from build123d import *

# Parameters (mm, degrees)
BOSS_EXTRUDE1_DEPTH                  = 3.175
F_1_4_0_25_DIAMETER_HOLE1_D          = 6.35
F_1_4_0_25_DIAMETER_HOLE3_AT_2_COUNT = 2
F_1_4_0_25_DIAMETER_HOLE3_AT_2_PITCH = 25.4
F_1_4_0_25_DIAMETER_HOLE3_AT_3_COUNT = 2
F_1_4_0_25_DIAMETER_HOLE3_AT_3_PITCH = 71.842048969
F_1_4_0_25_DIAMETER_HOLE3_AT_4_COUNT = 2
F_1_4_0_25_DIAMETER_HOLE3_AT_4_PITCH = 91.581002397


with BuildPart() as part:
    # Outline → Boss-Extrude1 (new body)
    with BuildSketch(Plane.XZ.offset(-43.833362877)):
        with BuildLine():
            Line((176.972439461, -654.113339272), (243.430903053, -587.760058499))
            ThreePointArc((243.430903053, -587.760058499), (244.176274012, -585.964597022), (243.433747886, -584.167957177))
            Line((243.433747886, -584.167957177), (231.320007239, -572.035013901))
            ThreePointArc((231.320007239, -572.035013901), (229.524545763, -571.289642942), (227.727905917, -572.032169067))
            Line((227.727905917, -572.032169067), (202.161954847, -597.557657288))
            ThreePointArc((202.161954847, -597.557657288), (175.212357167, -608.695549172), (148.280435018, -597.514984781))
            Line((148.280435018, -597.514984781), (123.155639602, -572.350361691))
            ThreePointArc((123.155639602, -572.350361691), (121.360178125, -571.604990731), (119.56353828, -572.347516857))
            Line((119.56353828, -572.347516857), (107.430595004, -584.461257504))
            ThreePointArc((107.430595004, -584.461257504), (106.685224045, -586.256718981), (107.42775017, -588.053358826))
            Line((107.42775017, -588.053358826), (173.380338139, -654.110494438))
            ThreePointArc((173.380338139, -654.110494438), (175.175799616, -654.855865397), (176.972439461, -654.113339272))
        make_face()
    extrude(amount=BOSS_EXTRUDE1_DEPTH)

    # 1/4 (0.25) Diameter Hole1 (through all)
    with Locations(Plane(origin=(0, 40.658362877, 0), x_dir=(-1, 0, 0), z_dir=(0, -1, 0))):
        with Locations((-175.18563451, 642.437587559), (-193.160365289, 624.491305118), (-157.239352069, 624.46285678)):
            Hole(F_1_4_0_25_DIAMETER_HOLE1_D / 2)

    # Sketch11 → 1/4 (0.25) Diameter Hole3 (revolve, cut)
    with BuildSketch(Plane(origin=(139.293069629, 40.658362877, -606.488126001), x_dir=(0, 0, -1), z_dir=(1, 0, 0))):
        Polygon((0, 0), (0, 3.175), (3.175, 3.175), (3.175, 3.944613268), (6.604, 0), align=None)
    f_1_4_0_25_diameter_hole3 = revolve(axis=Axis((139.293069629, 34.308362877, -606.488126001), (0, 1, 0)), mode=Mode.SUBTRACT)

    # 1/4 (0.25) Diameter Hole3 at 2: 1/4 (0.25) Diameter Hole3 ×2
    with Locations(*[Vector(-0.7065465527738991, 0, 0.7076665660912065) * (i * F_1_4_0_25_DIAMETER_HOLE3_AT_2_PITCH) for i in range(1, F_1_4_0_25_DIAMETER_HOLE3_AT_2_COUNT)]):
        add(f_1_4_0_25_diameter_hole3, mode=Mode.SUBTRACT)

    # 1/4 (0.25) Diameter Hole3 at 3: 1/4 (0.25) Diameter Hole3 ×2
    with Locations(*[Vector(0.9999996863924931, 0, -0.0007919690116880901) * (i * F_1_4_0_25_DIAMETER_HOLE3_AT_3_PITCH) for i in range(1, F_1_4_0_25_DIAMETER_HOLE3_AT_3_COUNT)]):
        add(f_1_4_0_25_diameter_hole3, mode=Mode.SUBTRACT)

    # 1/4 (0.25) Diameter Hole3 at 4: 1/4 (0.25) Diameter Hole3 ×2
    with Locations(*[Vector(0.980735686075181, 0, 0.1953394841260828) * (i * F_1_4_0_25_DIAMETER_HOLE3_AT_4_PITCH) for i in range(1, F_1_4_0_25_DIAMETER_HOLE3_AT_4_COUNT)]):
        add(f_1_4_0_25_diameter_hole3, mode=Mode.SUBTRACT)


solid = part.part
Geometry: final body of the model. Coordinates: model frame, mm. A direction names the side the tool comes from. Give positions to 0.01 mm unless a question says otherwise; leave off trailing zeros. Write each loop counter-clockwise with the first axis right and the second up, starting at its lowest first coordinate (ties: lowest second). Pieces come first, ordered by that corner, then holes.
(1) Cut plane C-C, the plane x = 130. Return loops of the section in (y, z), then the cut area to 3 significant figures.
(2) Cut plane A-A, the plane y = 41.4. Give the number of separate pieces and of enclosed holes in the cut face, then the cut area to 3 significant figures.
(3) Cut plane B-B, the plane z = -641. Return loops of the section in (x, y), then the cut area to 3 significant figures.
(4) Mould query, pull axis Z, two halves, no side actions, for faces 1 (the conical face through (227.903, 43.635, -592.43)), 2 (the cylindrical face through (175.148, 42.268, -654.856)), 3 (the cylindrical face through (192.75, 42.27, -627.64)), 4 (the cylindrical face through (121.388, 42.268, -571.605)). Classes: released by +Z, released by -Z, zero draft, split by the parting line, or undercut.
(5) Cut plane D-D, the plane z = -580. Return loops of the section in (x, y), then the cut area to 3 significant figures.
(6) Access query for faces 5 (the flat face through (135.894, 42.268, -585.109)), 6 (the conical face through (207.748, 43.635, -608.704)). Directions: +Z, -Z, +X, -X, +Y, -Y. A direction counts if a zero-diameter tool reaches every point of the face in a straight line with its end or side. Return the directions, or none.
(7) Ray query, line 1 (X direction, y = 43.5, z = -625); line 2 (X direction, y = 41.85, z = -600); line 3 (X direction, y = 41.85, z = -580). Return the intervals inside material, ascending.
(8) First-contact query: P1, Ø6, axis at x = 188.5, z = -602.5, coming from the -Y side; P2, Ø10, axis at x = 193.16, z = -624.49, coming from the -Y side; P3, Ø1, axis at y = 41.5, z = -597.5, coming from the -X side; P4, Ø1.5, axis at x = 126.5, y = 41, coming from the -Z side. Flat tips, straight axial feed; report the tip coordinate or a pass-through.
Values follow:
1. outline: (40.66, -610.66) - (43.83, -610.66) - (43.83, -579.21) - (40.66, -579.21) - close
1. area: 99.9 mm2
2. separate pieces: 1
2. enclosed holes: 7
2. area: 3,660 mm2
3. outline: (160.29, 40.66) - (172.35, 40.66) - (172.35, 43.83) - (160.29, 43.83) - close; (178.02, 40.66) - (190.11, 40.66) - (190.11, 43.83) - (178.02, 43.83) - close
3. area: 76.7 mm2
4. face 1: undercut
4. face 2: released by -Z
4. face 3: undercut
4. face 4: released by +Z
5. outline: (111.9, 40.66) - (130.79, 40.66) - (130.79, 43.83) - (111.9, 43.83) - close; (219.75, 40.66) - (239.27, 40.66) - (239.27, 43.83) - (219.75, 43.83) - close
5. area: 122 mm2
6. face 5: +Z, +Y, -Y
6. face 6: -Y
7. line 1: x = 144.32 to 154.11, 160.37 to 190.03, 196.29 to 206.13
7. line 2: x = 119.36 to 151.01, 199.47 to 231.17
7. line 3: x = 111.9 to 130.79, 219.75 to 239.27
8. P1: passes through
8. P2: stops at y = 40.66
8. P3: stops at x = 116.36
8. P4: stops at z = -607.91
